Can you work these out from the model? Positions are in its coordinate system, mm. A direction names the side the tool comes from. Coordinates: 2 decimals unless noted, no trailing zeros. Write each loop counter-clockwise with the first axis right and the second up, starting at its lowest first coordinate (ties: lowest second). Pieces come first, ordered by that corner, then holes. Notation, with made-up numbers: (-17, -14) - (9, -14) arc R22 cw to (9, 21) - close; hole circle Ø10 at (36.25, 70). An arc over 180 degrees is marked (long way). One line per question, with ' | ' between items. Start each with the question number.
from build123d import *

# Parameters (mm, degrees)
SKETCH_R   = 8.5
SKETCH_R_2 = 21.5
PAD_DEPTH  = 10


with BuildPart() as part:
    # Sketch → Pad (new body)
    with BuildSketch(Plane.XY):
        with BuildLine():
            ThreePointArc((-47.162932, -89.074877), (0, -146), (47.162932, -89.074877))
            ThreePointArc((77.017443, -12.861504), (51.124626, -46.672731), (47.162932, -89.074877))
            ThreePointArc((77.017443, -12.861504), (83.108641, 3.517146), (70.581481, 15.700461))
            Line((5.585185, 28.457085), (70.581481, 15.700461))
            ThreePointArc((5.585185, 28.457085), (0, 29), (-5.585185, 28.457085))
            Line((-5.585185, 28.457085), (-70.581481, 15.700461))
            ThreePointArc((-70.581481, 15.700461), (-83.108641, 3.517146), (-77.017443, -12.861504))
            ThreePointArc((-47.162932, -89.074877), (-51.124626, -46.672731), (-77.017443, -12.861504))
        make_face()
        with Locations((-67.5, 0)):
            Circle(SKETCH_R, mode=Mode.SUBTRACT)
        with Locations((67.5, 0)):
            Circle(SKETCH_R, mode=Mode.SUBTRACT)
        with Locations((0, -98)):
            Circle(SKETCH_R_2, mode=Mode.SUBTRACT)
        with BuildLine():
            ThreePointArc((9.337686, 3.578773), (0, 10), (-9.337686, 3.578773))
            ThreePointArc((-9.337686, 3.578773), (-14.420663, -22.367539), (-10.427083, -48.503704))
            ThreePointArc((-10.427083, -48.503704), (0, -56), (10.427083, -48.503704))
            ThreePointArc((10.427083, -48.503704), (14.420663, -22.367539), (9.337686, 3.578773))
        make_face(mode=Mode.SUBTRACT)
    extrude(amount=PAD_DEPTH)


solid = part.part
(1) If we section it at D-D on y = 0: List the corners of the cut face in (x, z) for me.
(2) If we section it at A-A on x = 0: List the corners of the cut face in (y, z) for me, plus the area to 3 significant figures.
(3) Which directions (+Z, -Z, +X, -X, +Y, -Y) give clear straight access to the entire face, cutting with the end or side of a thin tool? Please do faces 4 (the face through (14.428, -22.739, 4.93)), 5 (the face through (-37.628, 22.168, 4.93)).
(4) If we section it at B-B on y = -117.5: List the corners of the cut face in (x, z) for me, plus the area to 3 significant figures.
(5) If we section it at C-C on x = 67.5: List the corners of the cut face in (y, z) for me.
(6) If I drill on probe 1 along X at (y, z) = (6.5, 9.25); probe 2 along X at (y, z) = (-111.5, 3.75); probe 3 along X at (y, z) = (-45.5, 1.25), over which ranges is the centre line in solid material (lowest first)?
(7) I'm going to push a flat-ended pin straight in: pin 1 (3 mm diameter, centred on y = -40.5, z = 2, fed in from -X). Where does the tip first touch, or does it pass through?
(8) If we mould it in two halves opening along Y, with no side actions, what happens to faces 1 (the face through (-14.412, -21.996, 4.93)), 2 (the face through (0, 29, 5)), 3 (the face through (-1, -57, 0))? For each: +Y half, -Y half, draft (parallel to the pull), parting line (faces both ways), or undercut.
Values:
1) outline: (-83.5, 0) - (-76, 0) - (-76, 10) - (-83.5, 10) - close; (-59, 0) - (-10.61, 0) - (-10.61, 10) - (-59, 10) - close; (10.61, 0) - (59, 0) - (59, 10) - (10.61, 10) - close; (76, 0) - (83.5, 0) - (83.5, 10) - (76, 10) - close
2) outline: (-146, 0) - (-119.5, 0) - (-119.5, 10) - (-146, 10) - close; (-76.5, 0) - (-56, 0) - (-56, 10) - (-76.5, 10) - close; (10, 0) - (29, 0) - (29, 10) - (10, 10) - close | area: 660 mm2
3) face 4: +Z, -Z | face 5: +Z, -Z, -X, +Y
4) outline: (-43.86, 0) - (-9.06, 0) - (-9.06, 10) - (-43.86, 10) - close; (9.06, 0) - (43.86, 0) - (43.86, 10) - (9.06, 10) - close | area: 696 mm2
5) outline: (-21.2, 0) - (-8.5, 0) - (-8.5, 10) - (-21.2, 10) - close; (8.5, 0) - (16.31, 0) - (16.31, 10) - (8.5, 10) - close
6) probe 1: -82.12 to -72.98, -62.02 to -7.6, 7.6 to 62.02, 72.98 to 82.12 | probe 2: -46.06 to -16.73, 16.73 to 46.06 | probe 3: -51.6 to -11.37, 11.37 to 51.6
7) pin 1: x = -54.63
8) face 1: undercut | face 2: +Y half | face 3: draft
